```python
from build123d import *

# Parameters (mm, degrees)
BOSS_EXTRUDE1_DEPTH = 76.2
FILLET2_R           = 6.35


with BuildPart() as part:
    # Sketch2 → Boss-Extrude1 (new body)
    with BuildSketch(Plane.XY):
        with BuildLine():
            Line((61.468, 23.62454), (30.749865701, 23.62454))
            Line((30.749865701, 23.62454), (24.323763897, 21.014679926))
            ThreePointArc((24.323763897, 21.014679926), (23.327763264, 20.82831872), (22.338166155, 21.046138193))
            Line((22.338166155, 21.046138193), (11.472349033, 25.865540532))
            ThreePointArc((11.472349033, 25.865540532), (-23.719801629, -15.427637215), (28.2956, 0))
            Line((28.2956, 0), (28.2956, 18.01114))
            Line((28.2956, 18.01114), (61.468, 18.01114))
            Line((61.468, 18.01114), (61.468, 19.23034))
            Line((61.468, 19.23034), (27.0764, 19.23034))
            Line((27.0764, 19.23034), (27.0764, 0))
            ThreePointArc((27.0764, 0), (-22.697763498, -14.762891626), (10.978028787, 24.751046865))
            Line((10.978028787, 24.751046865), (21.843845909, 19.931644525))
            ThreePointArc((21.843845909, 19.931644525), (23.308449631, 19.609271705), (24.782530568, 19.88508629))
            Line((24.782530568, 19.88508629), (30.988, 22.40534))
            Line((30.988, 22.40534), (61.468, 22.40534))
            Line((61.468, 22.40534), (61.468, 23.62454))
        make_face()
    extrude(amount=BOSS_EXTRUDE1_DEPTH)

    # Fillet2
    fillet2_edges = [part.edges().sort_by_distance(p)[0] for p in [
        (61.468, 23.01494, 76.2),
        (61.468, 18.62074, 0),
        (61.468, 23.01494, 0),
        (61.468, 18.62074, 76.2),
    ]]
    fillet(fillet2_edges, radius=FILLET2_R)


solid = part.part
```
The model under review builds one solid part; all positions refer to its coordinate system, in mm. A direction names the side the tool comes from. Round coordinates to 2 decimals unless told otherwise and drop trailing zeros. Order: outer loops, then holes, each group sorted by start corner. A loop starts at its lowest first (then second) coordinate and runs counter-clockwise, first axis right, second up. Notation, with made-up numbers: (41.5, -18.75) -> (59.5, -18.75) arc R22 ccw to (59.5, 8.25) -> close; hole circle Ø3 at (-10, 70.5). An arc over 180 degrees is marked (long way). One line per item, written item: value. Start each with the question number.
Q1. Mouldability with a two-part tool opening along Y and no side actions: class faces 1 (the face through (16.335, 22.375, 37.567)), 2 (the face through (59.66, 23.02, 1.91)), 3 (the face through (16.981, 23.422, 37.567)) as released by +Y, released by -Y, zero draft, split by the parting line, or undercut.
Q2. Clearance check with flat-ended pins moving along their axes: pin 1 Ø15.5 at (y, z) = (13, 26.5) entering from -X; pin 2 Ø8 at (y, z) = (2, 39) entering from +X; pin 3 Ø1.5 at (x, z) = (1.5, 23) entering from +Y. State where each tip first meets the part, or that it passes through.
Q3. Take a section at C-C (y = -8). Write out the cut boundary in (x, z).
Q4. Take a section at A-A (x = 0). Write out the cut boundary in (y, z), and give its area (3 significant figures).
Q5. Take a section at B-B (z = 27.5). Write out the cut boundary in (x, y).
Q6. Wall thickness on line 1 (Y direction, x = 0, z = 38); line 2 (Y direction, x = 55, z = 47); line 3 (X direction, y = 0.5, z = 15): over which ranges is each line inside the solid? List them lowest first.
Q7. Machinability: for faces 4 (the face through (23.29, 19.61, 37.57)), 5 (the face through (27.842, 21.128, 37.567)), 6 (the face through (46, 23.625, 38)), which of the approach directions +Z, -Z, +X, -X, +Y, -Y give a long, thin tool a straight path to every point of the face, cutting with its end or side? Answer none if there is none.
Reported:
1. face 1: undercut
1. face 2: zero draft
1. face 3: released by +Y
2. pin 1: stops at x = -27.8
2. pin 2: stops at x = 28.3
2. pin 3: stops at y = 28.29
3. outline: (-27.14, 0) -> (-25.87, 0) -> (-25.87, 76.2) -> (-27.14, 76.2) -> close; (25.87, 0) -> (27.14, 0) -> (27.14, 76.2) -> (25.87, 76.2) -> close
4. outline: (-28.3, 0) -> (-27.08, 0) -> (-27.08, 76.2) -> (-28.3, 76.2) -> close; (27.08, 0) -> (28.3, 0) -> (28.3, 76.2) -> (27.08, 76.2) -> close
4. area: 186 mm2
5. outline: (10.98, 24.75) -> (21.84, 19.93) arc R3.76 ccw to (24.78, 19.89) -> (30.99, 22.41) -> (61.47, 22.41) -> (61.47, 23.62) -> (30.75, 23.62) -> (24.32, 21.01) arc R2.54 cw to (22.34, 21.05) -> (11.47, 25.87) arc R28.3 ccw (long way) to (28.3, 0) -> (28.3, 18.01) -> (61.47, 18.01) -> (61.47, 19.23) -> (27.08, 19.23) -> (27.08, 0) arc R27.08 cw (long way) to start
6. line 1: y = -28.3 to -27.08, 27.08 to 28.3
6. line 2: y = 18.01 to 19.23, 22.41 to 23.62
6. line 3: x = -28.29 to -27.07, 27.08 to 28.3
7. face 4: +Z, -Z
7. face 5: +Z, -Z, +X
7. face 6: +Z, -Z, +X, +Y
